Work out the finished part from the listing and answer in its coordinate system (mm). Face numbers are marked on the shaded views. Coordinates: 2 decimals unless noted, no trailing zeros. Write each loop counter-clockwise with the first axis right and the second up, starting at its lowest first coordinate (ties: lowest second). Pieces come first, ordered by that corner, then holes. Notation, with made-up numbers: (32, 32.25) - (60, 32.25) arc R18 ccw to (60, 55.25) - close; hole circle Ø5 at (75.25, -25.5). An arc over 180 degrees is marked (long way). One line per item, written item: value.
```python
from build123d import *

# Parameters (mm, degrees)
F0_R     = 12.7
F1_DEPTH = 12.7
F1_TAPER = 20
F2_R     = 3.175
F3_DEPTH = 101.6
F4_R     = 3.175
F5_DEPTH = 3.175
F5_TAPER = -7
F6_R     = 3.5648409809
F7_DEPTH = 17.78
F7_TAPER = 10
F8_W     = 15.24
F8_H     = 0.508
F9_DEPTH = 38.1


with BuildPart() as f1:
    # F0 (on Top) → F1 (new body)
    with BuildSketch(Plane.XY):
        Circle(F0_R)
    extrude(amount=F1_DEPTH, taper=F1_TAPER)

    # F2 (on face) → F3 (join)
    with BuildSketch(Plane.XY.offset(12.7)):
        Circle(F2_R)
    extrude(amount=F3_DEPTH)

    # F4 (on face) → F5 (join)
    with BuildSketch(Plane.XY.offset(114.3)):
        Circle(F4_R)
    extrude(amount=F5_DEPTH, taper=F5_TAPER)

    # F6 (on face) → F7 (join)
    with BuildSketch(Plane.XY.offset(117.475)):
        Circle(F6_R)
    extrude(amount=F7_DEPTH, taper=F7_TAPER)

    # F8 (on Top) → F9 (join)
    with BuildSketch(Plane.XY):
        Rectangle(F8_W, F8_H)
    extrude(amount=F9_DEPTH)

    # F10 (on Front) → F12 (revolve, cut)
    with BuildSketch(Plane.XZ):
        Polygon((-8.0804247409, 17.2624252737), (-3.1776875257, 38.326036185), (-8.6857005954, 39.8392230272), (-11.7726093158, 12.7228545025), (-3.1776875257, 12.7228545025), align=None)
    revolve(axis=Axis((0, 0, -4.9230908044), (0, 0, -1)), mode=Mode.SUBTRACT)


solid = f1.part
```
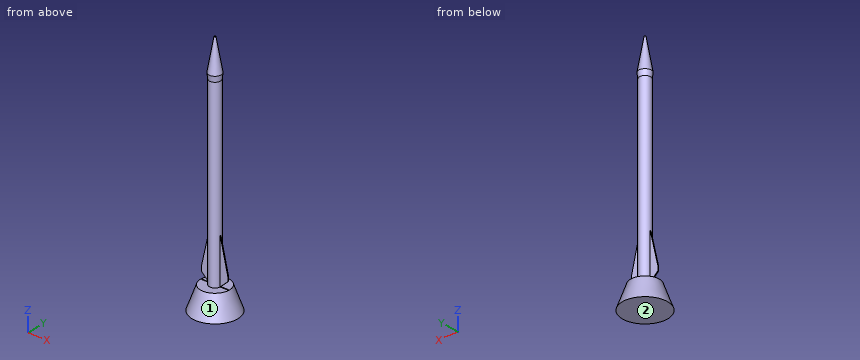
Item 1: Consider probe 1 along Y at (x, z) = (0, 14) (3 decimals); probe 2 along Y at (x, z) = (5, 22.5); probe 3 along Z at (x, y) = (4.5, -5.25). Determine where each line is inside the solid, lowest interval first.
Evaluation:
probe 1: y = -3.175 to 3.175
probe 2: y = -0.25 to 0.25
probe 3: z = 0 to 12.7
Item 2: Determine the mould class of the marked faces 1 and 2 for opening direction Y: +Y half, -Y half, draft (parallel to the pull), parting line (faces both ways), or undercut.
Evaluation:
face 1: parting line
face 2: draft
Item 3: Given pin 1 (3 mm diameter, centred on y = 3.5, z = 24, fed in from -X); pin 2 (2 mm diameter, centred on x = -6, z = 20, fed in from -Y); pin 3 (3.5 mm diameter, centred on x = 5.5, z = 31, fed in from +Y); pin 4 (8 mm diameter, centred on x = -9, z = 33.5, fed in from -Y), each flat-ended and moving along its own axis, determine where each tip first touches the part or whether it passes through.
Evaluation:
pin 1: stops at x = -2.47
pin 2: stops at y = -0.25
pin 3: stops at y = 0.25
pin 4: passes through
Item 4: Section A-A, the plane z = 90.5 is taken. Determine the outline of the cut face in (x, y) (3 decimals).
Evaluation:
outline: circle Ø6.35 at (0, 0)
